from build123d import *

# Parameters (mm, degrees)
F1_DEPTH = 2
F2_DEPTH = 16


with BuildPart() as f1:
    # F0 (on Top) → F1 (new body)
    with BuildSketch(Plane.XY):
        with BuildLine():
            ThreePointArc((13, 0), (3.628848584, 12.4832470918), (-10.9740704545, 6.969202082))
            ThreePointArc((-10.9740704545, 6.969202082), (-3.628848584, -12.4832470918), (13, 0))
        make_face()
        with BuildLine():
            ThreePointArc((10, 0), (-2.7914219877, -9.6024977629), (-8.4415926573, 5.3609246784))
            ThreePointArc((-8.4415926573, 5.3609246784), (-5.7521539146, 8.1800198865), (-2.1895164333, 9.7573571108))
            ThreePointArc((-2.1895164333, 9.7573571108), (6.2491933746, 7.8068932468), (10, 0))
        make_face(mode=Mode.SUBTRACT)
    extrude(amount=F1_DEPTH)

    # F0 (on Top) → F2 (join)
    with BuildSketch(Plane.XY):
        with BuildLine():
            ThreePointArc((-1.3684477708, 6.0983481943), (2.2173687229, 5.8434387091), (5.0696124466, 3.6553426161))
            ThreePointArc((5.0696124466, 3.6553426161), (5.9475868128, 1.9206017558), (6.25, 0))
            ThreePointArc((6.25, 0), (-1.7446387423, -6.0015611018), (-5.2759954108, 3.350577924))
            Line((-5.2759954108, 3.350577924), (-8.4415926573, 5.3609246784))
            ThreePointArc((-8.4415926573, 5.3609246784), (-2.7914219877, -9.6024977629), (10, 0))
            ThreePointArc((10, 0), (6.2491933746, 7.8068932468), (-2.1895164333, 9.7573571108))
            Line((-2.1895164333, 9.7573571108), (-1.3684477708, 6.0983481943))
        make_face()
        with BuildLine():
            Line((-8.4415926573, 5.3609246784), (-5.2759954108, 3.350577924))
            ThreePointArc((-5.2759954108, 3.350577924), (-3.5950961966, 5.112512429), (-1.3684477708, 6.0983481943))
            Line((-1.3684477708, 6.0983481943), (-2.1895164333, 9.7573571108))
            ThreePointArc((-2.1895164333, 9.7573571108), (-5.7521539146, 8.1800198865), (-8.4415926573, 5.3609246784))
        make_face()
    extrude(amount=F2_DEPTH)


solid = f1.part
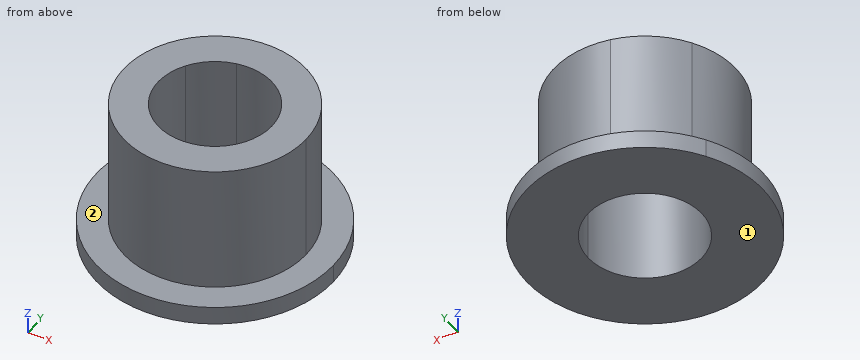
Can you work these out from the model? Positions are in its coordinate system, mm. Face numbers are marked on the shaded views. A direction names the side the tool comes from. Give positions to 0.01 mm unless a question says otherwise; leave off trailing zeros. Order: outer loops, then holes, each group sorted by start corner. A loop starts at its lowest first (then second) coordinate and runs counter-clockwise, first axis right, second up. Notation, with made-up numbers: M -18.5,73.25 L -9.5,73.25 A26 cw -9.5,90.25 Z; hole C 16.25,-0.5 d11. An arc over 180 degrees is marked long. One line per question, with ' | ' between items.
Item 1: Suppose I cut it at B-B, the plane z = 7.25. Write out the boundary of the cut face in (x, y), then the cut area to 3 significant figures.
Answer block:
outline: C 0,0 d20; hole C 0,0 d12.5 | area: 191 mm2
Item 2: For the marked faces 1 and 2, which set-ups out of +Z, -Z, +X, -X, +Y, -Y let a thin tool reach every point of the face, with its end or its side?
Answer block:
face 1: -Z, +X, -X, +Y, -Y | face 2: +Z
Item 3: Suppose I cut it at C-C, the plane y = -3.25. Write out the boundary of the cut face in (x, z), then the cut area to 3 significant figures.
Answer block:
outline: M -12.59,0 L -5.34,0 L -5.34,16 L -9.46,16 L -9.46,2 L -12.59,2 Z; M 5.34,0 L 12.59,0 L 12.59,2 L 9.46,2 L 9.46,16 L 5.34,16 Z | area: 144 mm2
Item 4: I'm going to push flat-ended pins straight in: pin 1 Ø7.5 at (x, y) = (0, 0) entering from +Z; pin 2 Ø4 at (x, z) = (-6, 5) entering from -Y; pin 3 Ø4 at (x, z) = (0.5, 7.5) entering from +Y; pin 4 Ø8 at (x, z) = (2.5, 14) entering from -Y. Where does each tip first touch, or does it pass through?
Answer block:
pin 1: passes through | pin 2: stops at y = -9.17 | pin 3: stops at y = 10 | pin 4: stops at y = -10
Item 5: Please list where these lines run through material, in increasing order: L1, parallel to Y at x = 0, z = 7.75; L2, parallel to Y at x = 5.5, z = 6.25; L3, parallel to X at y = 5, z = 2.25.
Answer block:
L1: y = -10 to -6.25, 6.25 to 10 | L2: y = -8.35 to -2.97, 2.97 to 8.35 | L3: x = -8.66 to -3.75, 3.75 to 8.66
Item 6: Suppose I cut it at D-D, the plane x = -9. Write out the boundary of the cut face in (y, z), then the cut area to 3 significant figures.
Answer block:
outline: M -9.38,0 L 9.38,0 L 9.38,2 L 4.36,2 L 4.36,16 L -4.36,16 L -4.36,2 L -9.38,2 Z | area: 160 mm2
Item 7: Suppose I cut it at A-A, the plane x = 0. Write out the boundary of the cut face in (y, z), then the cut area to 3 significant figures.
Answer block:
outline: M -13,0 L -6.25,0 L -6.25,16 L -10,16 L -10,2 L -13,2 Z; M 6.25,0 L 13,0 L 13,2 L 10,2 L 10,16 L 6.25,16 Z | area: 132 mm2
